Work out the finished part from the listing and answer in its coordinate system (mm). A direction names the side the tool comes from. Round coordinates to 2 decimals unless told otherwise and drop trailing zeros. Loops run counter-clockwise (first coordinate to the right, second up) from the corner with the lowest first, then second, coordinate; pieces in that order, holes last. Notation, with made-up numbers: (31.25, 66) -> (42.25, 66) arc R10 ccw to (42.25, 84) -> close; hole circle Ø5 at (69.25, 30.25). An arc over 180 degrees is marked (long way). Use one line per item in the form item = value.
```python
from build123d import *

# Parameters (mm, degrees)
EXTRUDE_1_DEPTH     = 8
SKETCH_3_R          = 8
SKETCH_3_R_2        = 6
EXTRUDE_3_DEPTH     = 27
SKETCH_5_R          = 6
CUT_EXTRUDE_1_DEPTH = 38.762415177
SKETCH_6_R          = 2.4
CUT_EXTRUDE_2_DEPTH = 38.762415177
SKETCH_7_R          = 9
CUT_EXTRUDE_3_DEPTH = 1.5
SKETCH_8_R          = 1
CUT_EXTRUDE_4_DEPTH = 52.86520992


with BuildPart() as part:
    # 草图2 → 凸台-拉伸1 (new body)
    with BuildSketch(Plane.XY):
        with BuildLine():
            Line((-16, 13.601470509), (-16, -13.601470509))
            ThreePointArc((-16, -13.601470509), (0, -21), (16, -13.601470509))
            Line((16, -13.601470509), (16, 13.601470509))
            ThreePointArc((16, 13.601470509), (0, 21), (-16, 13.601470509))
        make_face()
    extrude(amount=EXTRUDE_1_DEPTH)

    # 草图3 → 凸台-拉伸3 (add)
    with BuildSketch(Plane.XY.offset(8)):
        Circle(SKETCH_3_R)
        Circle(SKETCH_3_R_2, mode=Mode.SUBTRACT)
    extrude(amount=EXTRUDE_3_DEPTH)

    # 草图5 → 切除-拉伸1 (cut, through all)
    with BuildSketch(Plane.XY.offset(8)):
        Circle(SKETCH_5_R)
    extrude(amount=-CUT_EXTRUDE_1_DEPTH, mode=Mode.SUBTRACT)

    # 草图6 → 切除-拉伸2 (cut, through all)
    with BuildSketch(Plane.XY.offset(8)):
        with Locations((0, 16)):
            Circle(SKETCH_6_R)
        with Locations((11.313708499, 11.313708499)):
            Circle(SKETCH_6_R)
        with Locations((11.313708499, -11.313708499)):
            Circle(SKETCH_6_R)
        with Locations((0, -16)):
            Circle(SKETCH_6_R)
        with Locations((-11.313708499, -11.313708499)):
            Circle(SKETCH_6_R)
        with Locations((-11.313708499, 11.313708499)):
            Circle(SKETCH_6_R)
    extrude(amount=-CUT_EXTRUDE_2_DEPTH, mode=Mode.SUBTRACT)

    # 草图7 → 切除-拉伸3 (cut)
    with BuildSketch(Plane(origin=(0, 0, 0), x_dir=(-1, 0, 0), z_dir=(0, 0, -1))):
        Circle(SKETCH_7_R)
    extrude(amount=-CUT_EXTRUDE_3_DEPTH, mode=Mode.SUBTRACT)

    # 草图8 → 切除-拉伸4 (cut, through all)
    with BuildSketch(Plane.ZY.offset(16)):
        with Locations(Location((3.040852045, 0, 0), (0, 0, 270))):
            Circle(SKETCH_8_R)
    extrude(amount=-CUT_EXTRUDE_4_DEPTH, mode=Mode.SUBTRACT)


solid = part.part
```
(1) For faces 4 (the cylindrical face through (1.29, 18.024, 4.056)), 5 (the flat face through (-2, -6, 1.5)), 6 (the flat face through (7, 5, 8)), determine the directions among +Z, -Z, +X, -X, +Y, -Y from which every point of the face is accessible in a straight line to the end or side of a thin tool.
Completed:
face_4 = +Z, -Z
face_5 = -Z
face_6 = +Z
(2) Find section A-A, the plane x = 0. Write down the section's boundary in (y, z), then the cut area to 3 significant figures.
Completed:
outline = (-21, 0) -> (-18.4, 0) -> (-18.4, 8) -> (-21, 8) -> close; (-13.6, 0) -> (-9, 0) -> (-9, 1.5) -> (-6, 1.5) -> (-6, 35) -> (-8, 35) -> (-8, 8) -> (-13.6, 8) -> close; (6, 1.5) -> (9, 1.5) -> (9, 0) -> (13.6, 0) -> (13.6, 8) -> (8, 8) -> (8, 35) -> (6, 35) -> close; (18.4, 0) -> (21, 0) -> (21, 8) -> (18.4, 8) -> close
area = 262 mm2
(3) Consider L1, parallel to X at y = 11, z = 6.5; L2, parallel to X at y = 0, z = 5.5; L3, parallel to Z at x = 6.5, y = -6.5. Determine where each line is inside the solid, lowest interval first.
Completed:
L1 = -16 to -13.69, -8.93 to 8.93, 13.69 to 16
L2 = -16 to -6, 6 to 16
L3 = 0 to 8
(4) Find section D-D, the plane z = 6. Write down the section's boundary in (x, y).
Completed:
outline = (-16, -13.6) arc R21 ccw to (16, -13.6) -> (16, 13.6) arc R21 ccw to (-16, 13.6) -> close; hole circle Ø4.8 at (-11.31, -11.31); hole circle Ø4.8 at (-11.31, 11.31); hole circle Ø12 at (0, 0); hole circle Ø4.8 at (0, -16); hole circle Ø4.8 at (0, 16); hole circle Ø4.8 at (11.31, -11.31); hole circle Ø4.8 at (11.31, 11.31)
(5) Find section C-C, the plane y = 0. Write down the section's boundary in (x, z), then the cut area to 3 significant figures.
Completed:
outline = (-16, 0) -> (-9, 0) -> (-9, 1.5) -> (-6, 1.5) -> (-6, 2.04) -> (-16, 2.04) -> close; (-16, 4.04) -> (-6, 4.04) -> (-6, 35) -> (-8, 35) -> (-8, 8) -> (-16, 8) -> close; (6, 1.5) -> (9, 1.5) -> (9, 0) -> (16, 0) -> (16, 2.04) -> (6, 2.04) -> close; (6, 4.04) -> (16, 4.04) -> (16, 8) -> (8, 8) -> (8, 35) -> (6, 35) -> close
area = 219 mm2
(6) Find section B-B, the plane y = 16. Write down the section's boundary in (x, z), then the cut area to 3 significant figures.
Completed:
outline = (-13.6, 0) -> (-2.4, 0) -> (-2.4, 8) -> (-13.6, 8) -> close; (2.4, 0) -> (13.6, 0) -> (13.6, 8) -> (2.4, 8) -> close
area = 179 mm2
(7) For a pull along X with two mould halves and no side action, classify faces 1 (the flat face through (-16, 0, 5)), 2 (the cylindrical face through (1.172, 8.923, 0.74)), 3 (the flat face through (-2, 6, 35)) as +X half, -X half, draft (parallel to the pull), parting line (faces both ways), or undercut.
Completed:
face_1 = -X half
face_2 = undercut
face_3 = draft
(8) Given P1, Ø7.5, axis at x = -11.31, y = 11.31, coming from the +Z side; P2, Ø1.5, axis at x = 7, z = 27.5, coming from the +Y side; P3, Ø2, axis at y = 2, z = 18, coming from the -X side, each flat-ended and moving along its own axis, determine where each tip first touches the part or whether it passes through.
Completed:
P1 = 8
P2 = 4.99
P3 = -7.94
